from build123d import *

# Parameters (mm, degrees)
SKETCH1_R           = 1.5
BOSS_EXTRUDE2_DEPTH = 3.8
SKETCH2_W           = 3.5
SKETCH2_H           = 7
SKETCH2_H_2         = 5
BOSS_EXTRUDE3_DEPTH = 3.8
CUT_EXTRUDE1_DEPTH  = 2.3
SKETCH4_W           = 3.5
SKETCH4_H           = 7
CUT_EXTRUDE2_DEPTH  = 1.5
FILLET1_R           = 4


with BuildPart() as part:
    # Sketch1 → Boss-Extrude2 (new body)
    # profile 1 of 5: a face of its own
    with BuildSketch(Plane(origin=(0, 0, 0), x_dir=(1, 0, 0), z_dir=(0, 1, 0))):
        with BuildLine():
            Line((-11.834936491, -1.25), (-11.834936491, 1.25))
            ThreePointArc((-11.834936491, 1.25), (-16.5, 0), (-11.834936491, -1.25))
        make_face()
        with Locations(Location((-14, 0, 0), (0, 0, 90))):
            Circle(SKETCH1_R, mode=Mode.SUBTRACT)
    # profile 2 of 5: a face of its own
    with BuildSketch(Plane(origin=(0, 0, 0), x_dir=(1, 0, 0), z_dir=(0, 1, 0))):
        with BuildLine():
            ThreePointArc((-11.5, 0), (-11.585185434, 0.647047613), (-11.834936491, 1.25))
            Line((-11.834936491, 1.25), (-11.834936491, -1.25))
            ThreePointArc((-11.834936491, -1.25), (-11.585185434, -0.647047613), (-11.5, 0))
        make_face()
    # profile 3 of 5: a face of its own
    with BuildSketch(Plane(origin=(0, 0, 0), x_dir=(1, 0, 0), z_dir=(0, 1, 0))):
        with BuildLine():
            Line((11.834936491, 1.25), (-11.834936491, 1.25))
            ThreePointArc((-11.834936491, 1.25), (-11.585185434, 0.647047613), (-11.5, 0))
            ThreePointArc((-11.5, 0), (-11.585185434, -0.647047613), (-11.834936491, -1.25))
            Line((-11.834936491, -1.25), (11.834936491, -1.25))
            ThreePointArc((11.834936491, -1.25), (11.5, 0), (11.834936491, 1.25))
        make_face()
    # profile 4 of 5: a face of its own
    with BuildSketch(Plane(origin=(0, 0, 0), x_dir=(1, 0, 0), z_dir=(0, 1, 0))):
        with BuildLine():
            Line((11.834936491, -1.25), (11.834936491, 1.25))
            ThreePointArc((11.834936491, 1.25), (11.5, 0), (11.834936491, -1.25))
        make_face()
    # profile 5 of 5: a face of its own
    with BuildSketch(Plane(origin=(0, 0, 0), x_dir=(1, 0, 0), z_dir=(0, 1, 0))):
        with BuildLine():
            ThreePointArc((16.5, 0), (14.647047613, 2.414814566), (11.834936491, 1.25))
            Line((11.834936491, 1.25), (11.834936491, -1.25))
            ThreePointArc((11.834936491, -1.25), (14.647047613, -2.414814566), (16.5, 0))
        make_face()
        with Locations(Location((14, 0, 0), (0, 0, 90))):
            Circle(SKETCH1_R, mode=Mode.SUBTRACT)
    extrude(amount=BOSS_EXTRUDE2_DEPTH)

    # Sketch2 → Boss-Extrude3 (add)
    with BuildSketch(Plane(origin=(0, 3.8, 0), x_dir=(1, 0, 0), z_dir=(0, 1, 0))):
        with Locations((-3.25, 9.75)):
            Rectangle(SKETCH2_W, SKETCH2_H)
        with Locations((-3.25, 3.75)):
            Rectangle(SKETCH2_W, SKETCH2_H_2)
        with Locations((3.25, -3.75)):
            Rectangle(SKETCH2_W, SKETCH2_H_2)
        with Locations((3.25, -9.75)):
            Rectangle(SKETCH2_W, SKETCH2_H)
    extrude(amount=-BOSS_EXTRUDE3_DEPTH)

    # Sketch3 → Cut-Extrude1 (cut)
    with BuildSketch(Plane.XZ):
        with BuildLine():
            Line((5, 6.25), (1.5, 6.25))
            Line((1.5, 6.25), (1.5, 1.25))
            Line((1.5, 1.25), (-11.834936491, 1.25))
            ThreePointArc((-11.834936491, 1.25), (-11.5, 0), (-11.834936491, -1.25))
            Line((-11.834936491, -1.25), (-5, -1.25))
            Line((-5, -1.25), (-5, -6.25))
            Line((-5, -6.25), (-1.5, -6.25))
            Line((-1.5, -6.25), (-1.5, -1.25))
            Line((-1.5, -1.25), (11.834936491, -1.25))
            ThreePointArc((11.834936491, -1.25), (11.5, 0), (11.834936491, 1.25))
            Line((11.834936491, 1.25), (5, 1.25))
            Line((5, 1.25), (5, 6.25))
        make_face()
    extrude(amount=-CUT_EXTRUDE1_DEPTH, mode=Mode.SUBTRACT)

    # Sketch4 → Cut-Extrude2 (cut)
    with BuildSketch(Plane.XZ):
        with Locations((-3.25, -9.75)):
            Rectangle(SKETCH4_W, SKETCH4_H)
        with Locations((3.25, 9.75)):
            Rectangle(SKETCH4_W, SKETCH4_H)
    extrude(amount=-CUT_EXTRUDE2_DEPTH, mode=Mode.SUBTRACT)

    # Fillet1
    # the kernel refuses this fillet: 4 mm, written as the material it adds along each edge
    with BuildSketch(Plane(origin=(11.834936491, 2.3, -1.25), x_dir=(-1, 0, 0), z_dir=(0, 1, 0))) as fillet1_piece_1:
        with BuildLine():
            CenterArc((1.66736392, -4), FILLET1_R, 90, 36.128927472)
            ThreePointArc((-0.69105296, -0.769230769), (-0.305320518, -0.420735169), (0, 0))
            Line((0, 0), (1.66736392, 0))
        make_face()
    extrude(amount=1.5)
    with BuildSketch(Plane(origin=(-11.834936491, 2.3, 1.25), x_dir=(-0.668294067479168, 0, 0.743897196776644), z_dir=(0, 1, 0))) as fillet1_piece_2:
        with BuildLine():
            CenterArc((1.861299371, 3.913523616), FILLET1_R, 221.935536264, 36.128927472)
            Line((-1.114289416, 1.240347346), (0, 0))
            ThreePointArc((0, 0), (0.517027603, 0.05404774), (1.034055206, 0))
        make_face()
    extrude(amount=1.5)
    with BuildSketch(Plane(origin=(1.5, 3.8, 1.25), x_dir=(-1, 0, 0), z_dir=(0, -1, 0)), Plane(origin=(5, 3.8, 1.25), x_dir=(0, 0, 1), z_dir=(0, -1, 0))) as fillet1_piece_3:
        with BuildLine():
            CenterArc((FILLET1_R, -FILLET1_R), FILLET1_R, 90, 90)
            Line((0, -FILLET1_R), (0, 0))
            Line((0, 0), (FILLET1_R, 0))
        make_face()
    extrude(amount=1.5)
    with BuildSketch(Plane(origin=(-5, 3.8, -1.25), x_dir=(-1, 0, 0), z_dir=(0, -1, 0)), Plane(origin=(-1.5, 3.8, -1.25), x_dir=(0, 0, -1), z_dir=(0, -1, 0))) as fillet1_piece_4:
        with BuildLine():
            CenterArc((FILLET1_R, FILLET1_R), FILLET1_R, 180, 90)
            Line((0, FILLET1_R), (0, 0))
            Line((0, 0), (FILLET1_R, 0))
        make_face()
    extrude(amount=1.5)


solid = part.part
Build history of the part. All positions in model axes, mm. A direction names the side the tool comes from. Coordinates: 2 decimals unless noted, no trailing zeros. Order: outer loops, then holes, each group sorted by start corner. A loop starts at its lowest first (then second) coordinate and runs counter-clockwise, first axis right, second up. Notation, with made-up numbers: (37.25, 69) - (45.25, 69) arc R29 ccw to (45.25, 104) - close; hole circle Ø10 at (46.5, -5). An arc over 180 degrees is marked (long way). Write item = value, one per line. Start each with the question number.
1) Saw through at C-C on y = 3.4. Write the cut outline in (x, z).
2) Flat gauge pins, fed straight in: pin 1 Ø0.8 at (x, y) = (-10, 3) entering from -Z; pin 2 Ø2 at (y, z) = (0.5, 5) entering from -X; pin 3 Ø0.9 at (x, y) = (-3.5, 2) entering from +Z; pin 4 Ø1.2 at (y, z) = (2.5, -10) entering from +X. Where does each tip first touch, or does it go through?
3) Saw through at A-A on y = 0.65. Write the cut outline in (x, z).
4) 3-axis set-ups, long thin cutter, end or side, ignore diameter. For faces 1 (the face through (5, 3, 9)), 2 (the face through (-10, 3, -1.25)), 3 (the face through (10, 3, 1.25)): which of +Z, -Z, +X, -X, +Y, -Y reach the whole face in a straight line?
5) Saw through at B-B on x = 14. Write the cut outline in (y, z).
6) Wall check: line 1 along X through (y, z) = (1.35, 0); line 2 along X through (y, z) = (2.55, 0); line 3 along Z through (x, y) = (-14, 2). Give the ranges that are in metal, low to high. Write a range as from..to.
7) Saw through at D-D on x = -13. Write the cut outline in (y, z).
From the geometry:
q1.outline = (-12.53, 2.02) arc R2.5 ccw (long way) to (-11.83, -1.25) - (-9, -1.25) arc R4 cw to (-5, -5.25) - (-5, -13.25) - (-1.5, -13.25) - (-1.5, -5.25) arc R4 cw to (2.5, -1.25) - (10.17, -1.25) arc R4 cw to (12.53, -2.02) arc R2.5 ccw (long way) to (11.83, 1.25) - (9, 1.25) arc R4 cw to (5, 5.25) - (5, 13.25) - (1.5, 13.25) - (1.5, 5.25) arc R4 cw to (-2.5, 1.25) - (-10.17, 1.25) arc R4 cw to start; hole circle Ø3 at (-14, 0); hole circle Ø3 at (14, 0)
q2.pin_1 = -1.25
q2.pin_2 = through
q2.pin_3 = 1.25
q2.pin_4 = -1.5
q3.outline = circle Ø5 at (-14, 0); circle Ø5 at (14, 0); hole circle Ø3 at (-14, 0); hole circle Ø3 at (14, 0)
q4.face_1 = +Z, +X, +Y, -Y
q4.face_2 = -Z, +Y, -Y
q4.face_3 = +Z, +Y, -Y
q5.outline = (0, -2.5) - (3.8, -2.5) - (3.8, -1.5) - (0, -1.5) - close; (0, 1.5) - (3.8, 1.5) - (3.8, 2.5) - (0, 2.5) - close
q6.line_1 = -16.5..-15.5, -12.5..-11.5, 11.5..12.5, 15.5..16.5
q6.line_2 = -16.5..-15.5, -12.5..12.5, 15.5..16.5
q6.line_3 = -2.5..-1.5, 1.5..2.5
q7.outline = (0, -2.29) - (3.8, -2.29) - (3.8, -1.12) - (0, -1.12) - close; (0, 1.12) - (3.8, 1.12) - (3.8, 2.29) - (0, 2.29) - close
